Verification items for this drawing (mm, ordinates from the low corner). Give positions to 0.01 mm unless a question says otherwise; leave off trailing zeros. Order: outer loops, then holes, each group sorted by start corner. A loop starts at its lowest first (then second) coordinate and runs counter-clockwise, first axis right, second up.
(1) Scan lines: L1, parallel to Z at x = 11.25, y = 2.25; L2, parallel to Y at x = 8.5, z = 1; L3, parallel to X at y = 5.5, z = 1.55. Record each from-to range of solid material in increasing order.
(2) Sectioned sample at A-A on x = 12. Record the cut outline in (y, z), plus the area to 3 significant figures.
(3) Sectioned sample at B-B on z = 1.05. Record the cut outline in (x, y), plus the area to 3 significant figures.
(4) Gauge pin test, flat ends, axial feed: pin 1 (3 mm diameter, centred on x = 11, y = 4.5, fed in from -Z); pin 2 (1.5 mm diameter, centred on x = 7.5, z = 3.5, fed in from -Y); pin 3 (0.8 mm diameter, centred on x = 10.5, y = 2, fed in from +Z). Record the tip position at first contact, or that the pin passes through.
(5) Sectioned sample at D-D on z = 2.9. Record the cut outline in (x, y), plus the area to 3 significant figures.
(6) Sectioned sample at C-C on y = 6.25. Record the cut outline in (x, z).
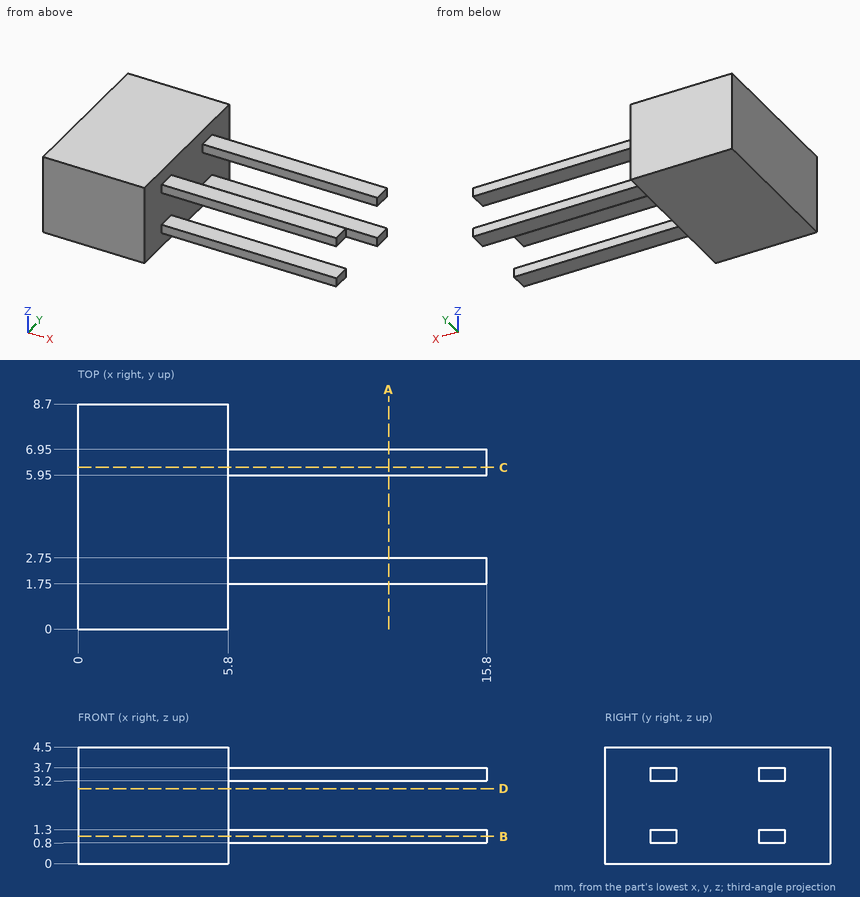
Ans:
1. L1: z = 0.8 to 1.3, 3.2 to 3.7
1. L2: y = 1.75 to 2.75, 5.95 to 6.95
1. L3: x = 0 to 5.8
2. outline: (1.75, 0.8) - (2.75, 0.8) - (2.75, 1.3) - (1.75, 1.3) - close; (1.75, 3.2) - (2.75, 3.2) - (2.75, 3.7) - (1.75, 3.7) - close; (5.95, 0.8) - (6.95, 0.8) - (6.95, 1.3) - (5.95, 1.3) - close; (5.95, 3.2) - (6.95, 3.2) - (6.95, 3.7) - (5.95, 3.7) - close
2. area: 2.00 mm2
3. outline: (0, 0) - (5.8, 0) - (5.8, 1.75) - (15.8, 1.75) - (15.8, 2.75) - (5.8, 2.75) - (5.8, 5.95) - (15.8, 5.95) - (15.8, 6.95) - (5.8, 6.95) - (5.8, 8.7) - (0, 8.7) - close
3. area: 70.5 mm2
4. pin 1: stops at z = 0.8
4. pin 2: stops at y = 1.75
4. pin 3: stops at z = 3.7
5. outline: (0, 0) - (5.8, 0) - (5.8, 8.7) - (0, 8.7) - close
5. area: 50.5 mm2
6. outline: (0, 0) - (5.8, 0) - (5.8, 0.8) - (15.8, 0.8) - (15.8, 1.3) - (5.8, 1.3) - (5.8, 3.2) - (15.8, 3.2) - (15.8, 3.7) - (5.8, 3.7) - (5.8, 4.5) - (0, 4.5) - close
